Model file for the job. Use its own axes, mm. Coordinates: 2 decimals unless noted, no trailing zeros. Order: outer loops, then holes, each group sorted by start corner. A loop starts at its lowest first (then second) coordinate and runs counter-clockwise, first axis right, second up.
from build123d import *

# Parameters (mm, degrees)
F1_DEPTH = 200
F3_DEPTH = 10
F5_DEPTH = 10


with BuildPart() as f1:
    # F0 (on Top) → F1 (new body)
    with BuildSketch(Plane.XY):
        Polygon((2.4, 1.1429430888), (0, 1.1429430888), (-2.4, 1.1429430888), (-2.4, 6), (-3.7251238391, 6), (-3.7251238391, 0), (-3.7251238391, -6), (-2.4, -6), (-2.4, -1.1429430888), (0, -1.1429430888), (2.4, -1.1429430888), (2.4, -6), (3.7251238391, -6), (3.7251238391, 0), (3.7251238391, 6), (2.4, 6), align=None)
    extrude(amount=F1_DEPTH)

    # F2 (on face) → F3 (join)
    with BuildSketch(Plane.XY.offset(200)):
        Polygon((-2.4, -6), (-2.4, -1.1429430888), (-2.4, 1.1429430888), (-2.4, 6), (-3.7251238391, 6), (-3.7251238391, -6), align=None)
        Polygon((2.4, 1.1429430888), (2.4, -1.1429430888), (2.4, -6), (3.7251238391, -6), (3.7251238391, 6), (2.4, 6), align=None)
    extrude(amount=F3_DEPTH)

    # F4 (on face) → F5 (cut)
    with BuildSketch(Plane(origin=(0, 0, 0), x_dir=(1, 0, 0), z_dir=(0, 0, -1))):
        Polygon((2.4, 1.1429430888), (2.4, -1.1429430888), (2.4, -6), (3.7251238391, -6), (3.7251238391, 6), (2.4, 6), align=None)
        Polygon((-2.4, -6), (-2.4, -1.1429430888), (-2.4, 1.1429430888), (-2.4, 6), (-3.7251238391, 6), (-3.7251238391, -6), align=None)
    extrude(amount=-F5_DEPTH, mode=Mode.SUBTRACT)


solid = f1.part
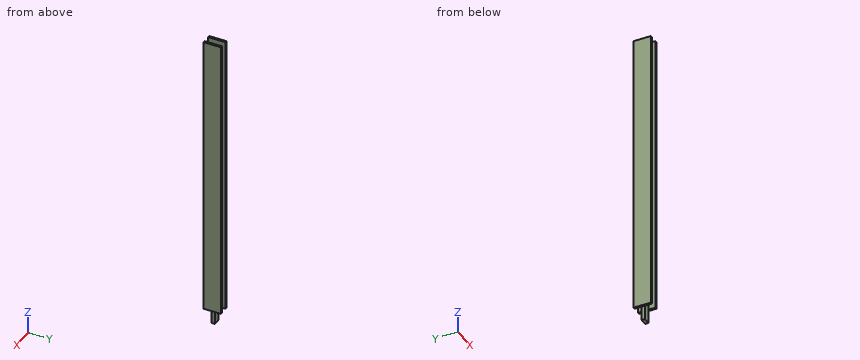
Q1. Cut at A-A, the plane y = -3.75. List the corners of the cut face in (x, z), plus the area to 3 significant figures.
Established:
outline: (-3.73, 10) - (-2.4, 10) - (-2.4, 210) - (-3.73, 210) - close; (2.4, 10) - (3.73, 10) - (3.73, 210) - (2.4, 210) - close
area: 530 mm2
Q2. Cut at B-B, the plane z = 123. List the corners of the cut face in (x, y), plus the area to 3 significant figures.
Established:
outline: (-3.73, -6) - (-2.4, -6) - (-2.4, -1.14) - (2.4, -1.14) - (2.4, -6) - (3.73, -6) - (3.73, 6) - (2.4, 6) - (2.4, 1.14) - (-2.4, 1.14) - (-2.4, 6) - (-3.73, 6) - close
area: 42.8 mm2
Q3. Probe line 1 (X direction, y = -5, z = 52); line 2 (Y direction, x = -1.75, z = 182.5); line 3 (Z direction, x = -0.75, y = -1). List the from-to ranges inside material, lowest first.
Established:
line 1: x = -3.73 to -2.4, 2.4 to 3.73
line 2: y = -1.14 to 1.14
line 3: z = 0 to 200
Q4. Cut at C-C, the plane x = 0. List the corners of the cut face in (y, z), plus the area to 3 significant figures.
Established:
outline: (-1.14, 0) - (1.14, 0) - (1.14, 200) - (-1.14, 200) - close
area: 457 mm2
Q5. Drop flat-ended pins along their axis: P1, Ø1.5, axis at x = 3, y = 1.5, coming from the -Z side; P2, Ø1.1, axis at y = -0.5, z = 7, coming from the +X side; P3, Ø2, axis at x = 0, z = 125, coming from the +Y side; P4, Ø1.8, axis at y = -0.5, z = 7.5, coming from the -X side. Give the stop position or say it passes through.
Established:
P1: stops at z = 0
P2: stops at x = 2.4
P3: stops at y = 1.14
P4: stops at x = -2.4
